CAD build for the part. Positions are in the model's coordinates, mm. A direction names the side the tool comes from. Give positions to 0.01 mm unless a question says otherwise; leave off trailing zeros. Write each loop counter-clockwise with the first axis right and the second up, starting at its lowest first coordinate (ties: lowest second). Pieces come first, ordered by that corner, then holes. Notation, with made-up numbers: M 1.25,29 L 59.25,29 A21 cw 59.25,40 Z; hole C 22,82 d9. An arc over 180 degrees is marked long. One line per question, with ' | ' between items. Start each with the question number.
1. Cut at C-C, the plane x = -3. Write the cut outline in (y, z).
2. Flat gauge pins, fed straight in: pin 1 (4 mm diameter, centred on x = -1.5, z = 0, fed in from +Y); pin 2 (6 mm diameter, centred on x = 2, z = 8, fed in from +Y); pin 3 (4 mm diameter, centred on x = -4, y = -8, fed in from -Z). Where does each tip first touch, or does it go through?
3. Wall check: L1, parallel to Z at x = 3.75, y = 0; L2, parallel to X at y = -3, z = -8.5. Give the ranges that are in metal, low to high.
4. Which spindle directions (+Z, -Z, +X, -X, +Y, -Y) get a long thin tool onto all of the face, cutting with end or side? Do faces 1 (the face through (8, 2, 7)), 2 (the face through (5, -8, -4)). Say none if no direction does.
5. Pull direction Y, two halves, no side cores. Call faces 3 (the face through (-7, 7, 0)), 4 (the face through (1, 0, -6)), 5 (the face through (6.49, -10.74, -2.38)): released by +Y, released by -Y, zero draft, split by the parting line, or undercut.
6. Cut at A-A, the plane y = 0. Write the cut outline in (x, z).
Solid Edge part; units mm, degrees
sketch "Sketch1" plane through (0, 0, 0) normal (0, -1, 0) x (1, 0, 0)
  line L0 (5, 11) -> (5, 8.5)
  line L1 (5, 8.5) -> (-7, 8.5)
  line L2 (-7, 8.5) -> (-7, 6)
  line L3 (-7, 6) -> (8, 6)
  line L4 (8, 6) -> (8, 11)
  line L5 (8, 11) -> (5, 11)
  dimension "D1" = 8
  dimension "D2" = 7
revolve "RevolvedProtrusion1" add sketch "Sketch1" angle 360 about axis through (0, 0, 0) along (1, 0, 0)
chamfer "Chamfer1" distance 0.8 angle 45 5 edges at (8, 0, -6) (8, 0, -11) (5, 0, -11) (-7, 0, -8.5) (-7, 0, -6)
properties part number "1976-1300-C05" material "Bronce, 90%"
Here are the results:
1) outline: C 0,0 d17; hole C 0,0 d12
2) pin 1: y = 8.5 | pin 2: y = 6.87 | pin 3: z = -6.02
3) L1: -8.5 to -6, 6 to 8.5 | L2: 5 to 8
4) face 1: +Z, -Z, +X, +Y, -Y | face 2: -X
5) face 3: zero draft | face 4: undercut | face 5: split by the parting line
6) outline: M -7,-7.7 L -6.2,-8.5 L 5,-8.5 L 5,-10.2 L 5.8,-11 L 7.2,-11 L 8,-10.2 L 8,-6.8 L 7.2,-6 L -6.2,-6 L -7,-6.8 Z; M -7,6.8 L -6.2,6 L 7.2,6 L 8,6.8 L 8,10.2 L 7.2,11 L 5.8,11 L 5,10.2 L 5,8.5 L -6.2,8.5 L -7,7.7 Z
